Verification items for the finished model (mm, model axes). A direction names the side the tool comes from. Give positions to 0.01 mm unless a question says otherwise; leave off trailing zeros. Order: outer loops, then holes, each group sorted by start corner. A loop starts at its lowest first (then second) coordinate and runs counter-clockwise, first axis right, second up. Notation, with made-up numbers: (71, 59.25) -> (113, 59.25) arc R25 cw to (113, 97.25) -> close; hole circle Ø1 at (77.25, -3). An arc over 180 degrees is marked (long way). One line per question, with ' | ' between items. Start each with the question number.
Q1. Mould release check, pull along Y, two halves, no side actions. Record for faces 1 (the flat face through (0, 1, 0)), 2 (the cylindrical face through (2.553, -3.613, 0.527)), 3 (the cylindrical face through (2.55, -3.24, 0.52)): released by +Y, released by -Y, zero draft, split by the parting line, or undercut.
Q2. Section check A-A on z = 0.25. Record the cut outline in (x, y).
Q3. Section check C-C on x = 2.5. Record the cut outline in (y, z), plus the area to 3 significant figures.
Q4. Section check B-B on y = 0. Record the cut outline in (x, z), plus the area to 3 significant figures.
Q5. Go/stop test with flat-tipped pins: pin 1 (1.5 mm diameter, centred on x = 3.5, y = -0.5, fed in from +Z); pin 2 (0.6 mm diameter, centred on x = 3, z = 1, fed in from +Y); pin 3 (0.8 mm diameter, centred on y = -3, z = 1, fed in from -X). Record where each tip stops, or that it passes through.
Q6. Section check D-D on z = 0.75. Record the cut outline in (x, y), plus the area to 3 significant figures.
Q7. Access from +Z, -Z, +X, -X, +Y, -Y to the whole of each face (thin tool, end or side, straight path). Record for faces 4 (the cylindrical face through (0.108, -0.488, 0.247)), 5 (the flat face through (0, 1, 0.5)).
Q8. Material ranges on probe 1 along Z at (x, y) = (4, 0); probe 2 along X at (y, z) = (-2.25, 1); probe 3 along Z at (x, y) = (2, -2.5), recorded low to high. Write a range as [from, to].
from build123d import *

# Parameters (mm, degrees)
F0_W      = 10.0359702483
F0_H      = 5.6423433125
F1_DEPTH  = 1
F2_R      = 0.7919203143
F3_DEPTH  = 10.55
F4_DEPTH  = 5
F5_R      = 0.4182620548
F6_DEPTH  = 25
F8_D      = 1
F8_DEPTH  = 2
F8_TIP    = 0.3004303095
F9_W      = 5.0282278639
F9_H      = 0.5
F10_DEPTH = 25


with BuildPart() as f1:
    # F0 (on Top) → F1 (new body)
    with BuildSketch(Plane.XY):
        Rectangle(F0_W, F0_H)
    extrude(amount=F1_DEPTH)

    # F2 (on face) → F3 (cut)
    with BuildSketch(Plane.YZ.offset(5.0179851241)):
        with Locations((-2.8211716563, 0.5)):
            Circle(F2_R)
    extrude(amount=-F3_DEPTH, mode=Mode.SUBTRACT)

    # F2 (on face) → F4 (join)
    with BuildSketch(Plane.YZ.offset(5.0179851241)):
        with Locations((-2.8211716563, 0.5)):
            Circle(F2_R)
    extrude(amount=-F4_DEPTH)

    # F5 (on face) → F6 (cut)
    with BuildSketch(Plane.YZ.offset(5.0179851241)):
        with Locations((-2.8211716563, 0.5)):
            Circle(F5_R)
    extrude(amount=-F6_DEPTH, mode=Mode.SUBTRACT)

    # F8
    with Locations(Plane.XY.offset(1)):
        with Locations((0, 0)):
            Hole(F8_D / 2, depth=F8_DEPTH)
            with Locations((0, 0, -(F8_DEPTH + F8_TIP / 2))):  # 118° drill point
                Cone(0, F8_D / 2, F8_TIP, mode=Mode.SUBTRACT)

    # F9 (on face) → F10 (cut)
    with BuildSketch(Plane.YZ.offset(5.0179851241)):
        with Locations((0.3070577243, 0.75)):
            Rectangle(F9_W, F9_H)
    extrude(amount=-F10_DEPTH, mode=Mode.SUBTRACT)


solid = f1.part
Filled in:
1) face 1: zero draft | face 2: split by the parting line | face 3: undercut
2) outline: (-5.02, -2.07) -> (0.02, -2.07) -> (0.02, -2.49) -> (5.02, -2.49) -> (5.02, 2.82) -> (-5.02, 2.82) -> close; (0.02, -3.57) -> (5.02, -3.57) -> (5.02, -3.16) -> (0.02, -3.16) -> close; hole circle Ø1 at (0, 0)
3) outline: (-2.21, 0) -> (2.82, 0) -> (2.82, 0.5) -> (-2.21, 0.5) -> (-2.21, 1) arc R0.79 ccw (long way) to start; hole circle Ø0.84 at (-2.82, 0.5) | area: 3.81 mm²
4) outline: (-5.02, 0) -> (-0.5, 0) -> (-0.5, 0.5) -> (-5.02, 0.5) -> close; (0.5, 0) -> (5.02, 0) -> (5.02, 0.5) -> (0.5, 0.5) -> close | area: 4.52 mm²
5) pin 1: z = 0.5 | pin 2: y = -2.21 | pin 3: x = 0.02
6) outline: (0.02, -3.57) -> (5.02, -3.57) -> (5.02, -3.16) -> (0.02, -3.16) -> close; (0.02, -2.49) -> (5.02, -2.49) -> (5.02, -2.21) -> (0.02, -2.21) -> close | area: 3.47 mm²
7) face 4: +Z, -Z | face 5: +Z, +X, -X, +Y
8) probe 1: [0, 0.5] | probe 2: [0.02, 5.02] | probe 3: [-0.22, 0.23], [0.77, 1.22]
